Autodesk Fusion 360 part; units mm, degrees
sketch "Sketch1" plane through (0, 0, 0) normal (0, 0, 1) x (1, 0, 0)
  line L0 (19.5, 10) -> (-19.5, 10)
  line L1 (-19.5, 10) -> (-19.5, -10)
  line L2 (-19.5, -10) -> (19.5, -10)
  line L3 (19.5, -10) -> (19.5, 10)
  line L4 (19.5, 10) -> (-19.5, -10) construction
  line L5 (-19.5, 10) -> (19.5, -10) construction
  circle A0 centre (0, 0) radius 2.6
  dimension "d1" = 5.2
  dimension "d2" = 39
  dimension "d3" = 20
extrude "Extrude1" add sketch "Sketch1" along normal blind 3.4
sketch "Sketch2" plane through (0, 0, 3.4) normal (0, 0, 1) x (-1, 0, 0)
  circle A0 centre (0, 0) radius 2.6
  line L0 (-19.5, 10) -> (-19.5, -10)
  line L1 (-19.5, -10) -> (19.5, -10)
  line L2 (19.5, -10) -> (19.5, 10)
  line L3 (19.5, 10) -> (-19.5, 10)
  line L4 (19.5, 3) -> (-19.5, 3)
  line L5 (19.5, -3) -> (-19.5, -3)
  line L6 (-19.5, 3) -> (19.5, -3) construction
  dimension "d7" = 6
extrude "Extrude2" add sketch "Sketch2" along normal blind 6 contours L0 L2 L4 L5
extrude "Extrude5" cut 1 faces at (-6.5, -10, 2.2667) along direction (0, 1, 0) up to surface (7 mm away)
sketch "Sketch3" plane through (0, 0, 9.4) normal (0, 0, 1) x (-1, 0, 0)
  line L0 (19.5, 3) -> (-19.5, 3)
  line L1 (-19.5, 3) -> (-19.5, -3)
  line L2 (-19.5, -3) -> (19.5, -3)
  line L3 (19.5, -3) -> (19.5, 3)
  line L4 (11, -3) -> (11, 3)
  line L5 (-11, -3) -> (-11, 3)
  circle A0 centre (0, 0) radius 2.6
  dimension "d11" = 11
  dimension "d12" = 11
extrude "Extrude3" cut sketch "Sketch3" against normal up to surface (6 mm away) contours L0 L2 L4 L5
extrude "Extrude4" cut 1 faces at (-16.6667, -3, 4.2667) along direction (0, 1, 0) blind 0.5
sketch "Sketch4" plane through (0, 0, 3.4) normal (0, 0, 1) x (-1, 0, 0)
  line L0 (11, 2.5) -> (0.7141, 2.5)
  arc A0 (-0.7141, 2.5) -> (0.7141, 2.5) centre (0, 0) ccw
  line L1 (-0.7141, 2.5) -> (-11, 2.5)
  line L2 (-11, 2.5) -> (-11, -3)
  line L3 (-11, -3) -> (-19.5, -3)
  line L4 (-19.5, -3) -> (-19.5, -10)
  line L5 (-19.5, -10) -> (19.5, -10)
  line L6 (19.5, -10) -> (19.5, -3)
  line L7 (19.5, -3) -> (11, -3)
  line L8 (11, -3) -> (11, 2.5)
  line L9 (10, -10) -> (13.5, -6.5)
  line L10 (13.5, -6.5) -> (19.5, -6.5)
  line L11 (-10, -10) -> (-13.5, -6.5)
  line L12 (-13.5, -6.5) -> (-19.5, -6.5)
  dimension "d24" = 20
  dimension "d25" = 3.5
  dimension "d26" = 3.5
  dimension "d27" = 135
  dimension "d28" = 135
extrude "Extrude6" cut sketch "Sketch4" against normal through all contours L5 L6 L9 L10 | L4 L5 L11 L12
fillet "Fillet2" radius 1 10 edges at (-19.5, -2.5, 4.7) (19.5, -2.5, 4.7) (11, 3, 6.4) (-11, 3, 6.4) (19.5, 6.5, 1.7) (-19.5, 6.5, 1.7) (-10, 10, 1.7) (10, 10, 1.7) (-13.5, 6.5, 1.7) (13.5, 6.5, 1.7)
fillet "Fillet1" radius 1 8 edges at (-15.25, -2.5, 9.4) (-19.5, 0.25, 9.4) (-11, 0.25, 9.4) (-15.25, 3, 9.4) (11, 0.25, 9.4) (15.25, -2.5, 9.4) (15.25, 3, 9.4) (19.5, 0.25, 9.4)
chamfer "Chamfer1" distance 0.5 angle 45 3 edges at (-19.5, 3.75, 0) (0, 10, 0) (19.5, 3.75, 0)
fillet "Fillet3" radius 0.5 2 edges at (-0.7141, -2.5, 1.95) (0.7141, -2.5, 1.95)
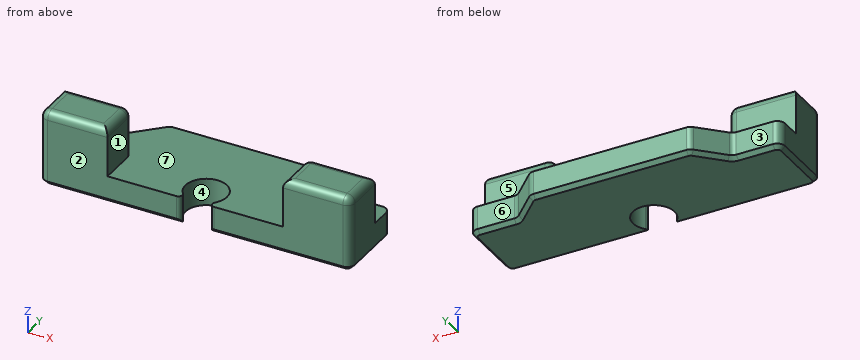
Model file for the job. Use its own axes, mm. Face numbers are marked on the shaded views. A direction names the side the tool comes from. Round coordinates to 2 decimals unless told otherwise and drop trailing zeros. Order: outer loops, then holes, each group sorted by start corner. A loop starts at its lowest first (then second) coordinate and runs counter-clockwise, first axis right, second up.
(1) Drill centre lines: line 1 (X direction, y = 0, z = 1.9); line 2 (X direction, y = 0, z = 5.5); line 3 (Z direction, x = 13, y = 5). Where is each one in solid material? Low to high.
(2) Pull direction Y, two halves, no side cores. Call the marked faces 1, 2, 3 and 4: released by +Y, released by -Y, zero draft, split by the parting line, or undercut.
(3) 3-axis set-ups, long thin cutter, end or side, ignore diameter. For the marked faces 5, 6 and 7: which of +Z, -Z, +X, -X, +Y, -Y reach the whole face in a straight line?
(4) Band-saw the part on C-C (x = 0). List the corners of the cut face in (y, z), then the cut area to 3 significant figures.
(5) Band-saw the part on A-A (z = 7). List the corners of the cut face in (x, y).
(6) Band-saw the part on B-B (y = 0). List the corners of the cut face in (x, z), then the cut area to 3 significant figures.
(7) Band-saw the part on D-D (z = 1.5). List the corners of the cut face in (x, y), then the cut area to 3 significant figures.
(8) Pin check, flat tips, straight feed: pin 1 (3 mm diameter, centred on x = -15.5, z = 1.5, fed in from +Y); pin 2 (1.5 mm diameter, centred on x = -15.5, z = 5, fed in from +Y); pin 3 (1 mm diameter, centred on x = -2.5, z = 4.5, fed in from +Y); pin 4 (4 mm diameter, centred on x = 14, y = 8.5, fed in from -Z). Stop position of each tip, or through.
Verdict:
1. line 1: x = -19.5 to -2.6, 2.6 to 19.5
1. line 2: x = -19.5 to -11, 11 to 19.5
1. line 3: z = 0 to 3.4
2. face 1: zero draft
2. face 2: released by -Y
2. face 3: released by +Y
2. face 4: undercut
3. face 5: +Z, +X, -X, +Y
3. face 6: +Z, -Z, +X, +Y
3. face 7: +Z, +Y
4. outline: (2.6, 0) - (9.5, 0) - (10, 0.5) - (10, 3.4) - (2.6, 3.4) - close
4. area: 25.0 mm2
5. outline: (-19.5, -1.5) arc R1 ccw to (-18.5, -2.5) - (-11, -2.5) - (-11, 2) arc R1 ccw to (-12, 3) - (-19.5, 3) - close; (11, -2.5) - (18.5, -2.5) arc R1 ccw to (19.5, -1.5) - (19.5, 3) - (12, 3) arc R1 ccw to (11, 2) - close
6. outline: (-19.5, 0.5) - (-19, 0) - (-2.6, 0) - (-2.6, 3.4) - (-11, 3.4) - (-11, 8.4) arc R1 ccw to (-12, 9.4) - (-18.5, 9.4) arc R1 ccw to (-19.5, 8.4) - close; (2.6, 0) - (19, 0) - (19.5, 0.5) - (19.5, 8.4) arc R1 ccw to (18.5, 9.4) - (12, 9.4) arc R1 ccw to (11, 8.4) - (11, 3.4) - (2.6, 3.4) - close
6. area: 216 mm2
7. outline: (-19.5, -1.5) arc R1 ccw to (-18.5, -2.5) - (-2.37, -2.5) arc R0.5 ccw to (-1.99, -1.68) arc R2.6 cw (long way) to (1.99, -1.68) arc R0.5 ccw to (2.37, -2.5) - (18.5, -2.5) arc R1 ccw to (19.5, -1.5) - (19.5, 5.5) arc R1 ccw to (18.5, 6.5) - (13.91, 6.5) arc R1 cw to (13.21, 6.79) - (10.29, 9.71) arc R1 ccw to (9.59, 10) - (-9.59, 10) arc R1 ccw to (-10.29, 9.71) - (-13.21, 6.79) arc R1 cw to (-13.91, 6.5) - (-18.5, 6.5) arc R1 ccw to (-19.5, 5.5) - close
7. area: 410 mm2
8. pin 1: stops at y = 6.5
8. pin 2: stops at y = 3
8. pin 3: passes through
8. pin 4: stops at z = 0.27
